Autodesk Inventor part; units mm, degrees
ref_plane "YZ Plane" through (0, 0, 0) normal (1, 0, 0) x (0, 1, 0)
ref_plane "XZ Plane" through (0, 0, 0) normal (0, 1, 0) x (-1, 0, 0)
ref_plane "XY Plane" through (0, 0, 0) normal (0, 0, 1) x (1, 0, 0)
sketch "Sketch1" plane through (0, 0, 0) normal (0, 1, 0) x (-1, 0, 0)
  line L0 (-4, 3.15) -> (4, 3.15)
  line L1 (4, 3.15) -> (4, -3.15)
  line L2 (4, -3.15) -> (-4, -3.15)
  line L3 (-4, -3.15) -> (-4, 3.15)
  line L4 (-4, 3.15) -> (4, -3.15) construction
  line L5 (4, 3.15) -> (-4, -3.15) construction
  line L6 (-2, 4) -> (2, 4)
  line L7 (2, 4) -> (2, -4)
  line L8 (2, -4) -> (-2, -4)
  line L9 (-2, -4) -> (-2, 4)
  line L10 (-2, 4) -> (2, -4) construction
  line L11 (2, 4) -> (-2, -4) construction
  line L12 (2, -4) -> (2.4907, -3.15)
  line L13 (2, -4) -> (2.9815, -4) construction
  line L14 (-2, -4) -> (-2.4907, -3.15)
  line L15 (-2, -4) -> (-1.0185, -4) construction
  line L16 (-2, 4) -> (-2.4907, 3.15)
  line L17 (-2, 4) -> (-1.0185, 4) construction
  line L18 (2, 4) -> (2.4907, 3.15)
  line L19 (2, 4) -> (2.9815, 4) construction
  point P0 (0, 0)
  dimension "d0" = 8
  dimension "d1" = 6.3
  dimension "d2" = 4
  dimension "d3" = 8
  dimension "d4" = 60
  dimension "d5" = 120
  dimension "d6" = 120
  dimension "d7" = 60
extrude "Extrusion1" add sketch "Sketch1" along normal blind 4.2
extrude "Extrusion2" cut sketch "Sketch1" along normal blind 3.5
extrude "Extrusion3" add sketch "Sketch1" along normal blind 0.8
sketch "Sketch2" plane through (0, 0.8, 0) normal (0, 1, 0) x (1, 0, 0)
  circle A0 centre (0, 0) radius 3
  dimension "d14" = 6
extrude "Extrusion4" add sketch "Sketch2" along normal up to next
properties part number "inductor"
Input: part model. Units: mm. Frame: model coordinates. Coordinates: 2 decimals unless noted, no trailing zeros. Order: outer loops, then holes, each group sorted by start corner. A loop starts at its lowest first (then second) coordinate and runs counter-clockwise, first axis right, second up. Notation, with made-up numbers: M 29,78.25 L 36,78.25 A17 ccw 36,85.25 Z; hole C 61.5,89.25 d1. An arc over 180 degrees is marked long. Write item = value, one per line. Start each with the question number.
(1) Section D-D on y = 2.25. Output: boundary loops of the cut face in (x, z).
(2) Section B-B on x = 3.5. Output: boundary loops of the cut face in (y, z), and give its area (3 significant figures).
(3) Section C-C on y = 0.35. Output: boundary loops of the cut face in (x, z), and give its area (3 significant figures).
(4) Pull-direction query (Y, two-part tool) for faces 1 (the flat face through (-2, 3.5, 3)), 2 (the flat face through (0, 4.2, 0)), 3 (the flat face through (-2, 0.8, 3)), 4 (the flat face through (0, 0, 0)); classes: released by +Y, released by -Y, zero draft, split by the parting line, or undercut.
(5) Section A-A on z = 0. Output: boundary loops of the cut face in (x, y).
(6) Line query: line 1 along Y through (x, z) = (-1, 3.25); line 2 along Z through (x, y) = (2.75, 3.7); line 3 along Z through (x, y) = (0, 2.45). Output: solid intervals per line, ascending. Write a range as [from, to].
(7) First-contact query: P1, Ø0.6, axis at x = -3.5, y = 0.5, coming from the -Z side; P2, Ø1, axis at y = 2.5, z = 1, coming from the -X side; P3, Ø0.6, axis at x = -3, y = 4, coming from the +Z side. Flat tips, straight axial feed; report the tip coordinate or a pass-through.
Result set:
q1.outline = C 0,0 d6
q2.outline = M 0,-3.15 L 0.8,-3.15 L 0.8,3.15 L 0,3.15 Z; M 3.5,-3.15 L 4.2,-3.15 L 4.2,3.15 L 3.5,3.15 Z
q2.area = 9.45 mm²
q3.outline = M -4,-3.15 L -2.49,-3.15 L -2,-4 L 2,-4 L 2.49,-3.15 L 4,-3.15 L 4,3.15 L 2.49,3.15 L 2,4 L -2,4 L -2.49,3.15 L -4,3.15 Z
q3.area = 58.0 mm²
q4.face_1 = undercut
q4.face_2 = released by +Y
q4.face_3 = undercut
q4.face_4 = released by -Y
q5.outline = M -4,0 L 4,0 L 4,0.8 L 3,0.8 L 3,3.5 L 4,3.5 L 4,4.2 L -4,4.2 L -4,3.5 L -3,3.5 L -3,0.8 L -4,0.8 Z
q6.line_1 = [0, 0.8], [3.5, 4.2]
q6.line_2 = [-3.15, 3.15]
q6.line_3 = [-3, 3]
q7.P1 = -3.15
q7.P2 = -2.96
q7.P3 = 3.15
